Autodesk Inventor part; units mm, degrees
ref_plane "YZ Plane" through (0, 0, 0) normal (1, 0, 0) x (0, 1, 0)
ref_plane "XZ Plane" through (0, 0, 0) normal (0, 1, 0) x (-1, 0, 0)
ref_plane "XY Plane" through (0, 0, 0) normal (0, 0, 1) x (1, 0, 0)
sketch "Boceto1" plane through (0, 0, 0) normal (0, 1, 0) x (-1, 0, 0)
  circle A0 centre (0, 0) radius 62
  dimension "d0" = 124
extrude "Extrusión1" add sketch "Boceto1" along normal blind 5
sketch "Boceto2" plane through (0, 5, 0) normal (0, 1, 0) x (1, 0, 0)
  circle A0 centre (0, 0) radius 41
  dimension "d3" = 82
extrude "Extrusión2" add sketch "Boceto2" along normal blind 11
sketch "Boceto3" plane through (0, 16, 0) normal (0, 1, 0) x (1, 0, 0)
  circle A0 centre (-32, 0) radius 5
  circle A1 centre (0, -32) radius 5
  circle A2 centre (32, 0) radius 5
  circle A3 centre (0, 32) radius 5
  point P0 (0, 0)
  dimension "d7" = 10
  dimension "d10" = 360
extrude "Extrusión3" cut sketch "Boceto3" against normal blind 4
sketch "Boceto4" plane through (32, 12, 0) normal (0, 1, 0) x (1, 0, 0)
  circle A0 centre (0, 0) radius 3.3
  circle A1 centre (-32, 32) radius 3.3
  circle A2 centre (-64, 0) radius 3.3
  circle A3 centre (-32, -32) radius 3.3
  point P0 (-32, 0)
  dimension "d14" = 6.6
  dimension "d17" = 360
extrude "Extrusión4" cut sketch "Boceto4" against normal blind 12
sketch "Boceto5" plane through (0, 0, 0) normal (0, -1, 0) x (1, 0, 0)
  circle A0 centre (0, 0) radius 21
  dimension "d21" = 42
extrude "Extrusión5" cut sketch "Boceto5" against normal blind 12
fillet "Empalme1" radius 2 1 edges at (-41, 16, 0)
fillet "Empalme2" radius 1 1 edges at (-21, 12, 0)
properties part number "Trabajo Dibujo pieza1"
Here's how the part is built. I have some questions about the finished solid (model axes, mm). A direction names the side the tool comes from. Give positions to 0.01 mm unless a question says otherwise; leave off trailing zeros. Order: outer loops, then holes, each group sorted by start corner. A loop starts at its lowest first (then second) coordinate and runs counter-clockwise, first axis right, second up. Notation, with made-up numbers: M -23,86.5 L 31,86.5 A31 cw 31,119.5 Z; hole C 51.5,49 d4. An arc over 180 degrees is marked long. Use a Markdown table: item, result. Add a question column.
1. Suppose I cut it at D-D (z = -51.5). List the corners of the cut face in (x, y) for me, and give its area (3 significant figures).
2. For pin 1 Ø3 at (x, y) = (-49.5, 5.5) entering from -Z; pin 2 Ø8.5 at (x, z) = (-32, 0) entering from +Y; pin 3 Ø8 at (x, y) = (-28.5, 10) entering from -Z, each with a flat end and sliding along its axis, tell me the tip position at first contact or that it passes through.
3. Suppose I cut it at C-C (y = 9.5). List the corners of the cut face in (x, z) for me, and give its area (3 significant figures).
4. I need wall thicknesses on probe 1 along Z at (x, y) = (0, 8.75); probe 2 along Z at (x, y) = (0, 14.25); probe 3 along Z at (x, y) = (0, 15.15). Which ranges of each line are inside material? Lowest first, please. Write a range as from..to.
5. Suppose I cut it at A-A (z = 0). Give the number of separate pieces and of enclosed holes in the cut face, and give its area (3 significant figures).
6. If we mould it in two halves opening along X, with no side actions, what happens to faces 4 (the cylindrical face through (-9, 9, -40)), 5 (the flat face through (-1.2, 12, 35.3)), 6 (the flat face through (-1, 16, -1))? For each: +X half, -X half, draft (parallel to the pull), parting line (faces both ways), or undercut.
7. On a 3-axis mill with a long thin cutter (end or side, diameter ignored), from which of +Z, -Z, +X, -X, +Y, -Y can I reach the whole of each face in a straight line? I mean faces 1 (the cylindrical face through (-1.08, 14.03, 36.88)), 2 (the cylindrical face through (-28.95, 6.08, 1.26)), 3 (the flat face through (0, 12, 0)). Say none if no direction works.
Results list:
| question | item | result |
|---|---|---|
| 1 | outline | M -34.52,0 L 34.52,0 L 34.52,5 L -34.52,5 Z |
| 1 | area | 345 mm² |
| 2 | pin 1 | stops at z = -39.14 |
| 2 | pin 2 | stops at y = 12 |
| 2 | pin 3 | stops at z = -32.87 |
| 3 | outline | C 0,0 d82; hole C -32,0 d6.6; hole C 0,0 d42; hole C 0,-32 d6.6; hole C 0,32 d6.6; hole C 32,0 d6.6 |
| 3 | area | 3,760 mm² |
| 4 | probe 1 | z = -41..-35.3, -28.7..-21, 21..28.7, 35.3..41 |
| 4 | probe 2 | z = -40.98..-37, -27..27, 37..40.98 |
| 4 | probe 3 | z = -40.64..-37, -27..27, 37..40.64 |
| 5 | separate pieces | 3 |
| 5 | enclosed holes | 0 |
| 5 | area | 778 mm² |
| 6 | face 4 | parting line |
| 6 | face 5 | undercut |
| 6 | face 6 | draft |
| 7 | face 1 | +Y |
| 7 | face 2 | +Y, -Y |
| 7 | face 3 | -Y |
